Geometry: final body of the model. Coordinates: model frame, mm. Face numbers are marked on the shaded views. A direction names the side the tool comes from. Give positions to 0.01 mm unless a question says otherwise; leave off trailing zeros. Loops run counter-clockwise (first coordinate to the right, second up) from the corner with the lowest first, then second, coordinate; pieces in that order, holes last. Notation, with made-up numbers: (25, 10.5) - (29, 10.5) arc R15 ccw to (29, 27.5) - close; hole circle Ø6 at (-20.5, -34). An arc over 180 degrees is marked (long way). Use one line per item in the form item = value.
```python
from build123d import *

# Parameters (mm, degrees)
F0_R     = 6.985
F1_DEPTH = 12.7


with BuildPart() as f1:
    # F0 (on Top) → F1 (new body)
    with BuildSketch(Plane.XY):
        with BuildLine():
            ThreePointArc((-3.175, 9.651164), (0, 10.16), (3.175, 9.651164))
            Line((3.175, 9.651164), (3.175, 24.243791))
            Line((3.175, 24.243791), (1.5875, 24.243791))
            Line((1.5875, 24.243791), (1.5875, 11.548717))
            Line((1.5875, 11.548717), (-1.5875, 11.548717))
            Line((-1.5875, 11.548717), (-1.5875, 24.243791))
            Line((-1.5875, 24.243791), (-3.175, 24.243791))
            Line((-3.175, 24.243791), (-3.175, 9.651164))
        make_face()
        with BuildLine():
            Line((3.175, 7.733791), (3.175, 9.651164))
            ThreePointArc((3.175, 9.651164), (0, 10.16), (-3.175, 9.651164))
            Line((-3.175, 9.651164), (-3.175, 7.733791))
            Line((-3.175, 7.733791), (3.175, 7.733791))
        make_face()
        with BuildLine():
            Line((7.733791, 3.175), (9.651164, 3.175))
            ThreePointArc((9.651164, 3.175), (7.184205, 7.184205), (3.175, 9.651164))
            Line((3.175, 9.651164), (3.175, 7.733791))
            Line((3.175, 7.733791), (-3.175, 7.733791))
            Line((-3.175, 7.733791), (-3.175, 9.651164))
            ThreePointArc((-3.175, 9.651164), (-7.184205, 7.184205), (-9.651164, 3.175))
            Line((-9.651164, 3.175), (-7.733791, 3.175))
            Line((-7.733791, 3.175), (-7.733791, -3.175))
            Line((-7.733791, -3.175), (-9.651164, -3.175))
            ThreePointArc((-9.651164, -3.175), (-7.184205, -7.184205), (-3.175, -9.651164))
            Line((-3.175, -9.651164), (-3.175, -7.733791))
            Line((-3.175, -7.733791), (3.175, -7.733791))
            Line((3.175, -7.733791), (3.175, -9.651164))
            ThreePointArc((3.175, -9.651164), (7.184205, -7.184205), (9.651164, -3.175))
            Line((9.651164, -3.175), (7.733791, -3.175))
            Line((7.733791, -3.175), (7.733791, 3.175))
        make_face()
        Circle(F0_R, mode=Mode.SUBTRACT)
        with BuildLine():
            ThreePointArc((9.651164, -3.175), (10.031985, -1.607758), (10.16, 0))
            ThreePointArc((10.16, 0), (10.031985, 1.607758), (9.651164, 3.175))
            Line((9.651164, 3.175), (7.733791, 3.175))
            Line((7.733791, 3.175), (7.733791, -3.175))
            Line((7.733791, -3.175), (9.651164, -3.175))
        make_face()
        with BuildLine():
            ThreePointArc((9.651164, 3.175), (10.031985, 1.607758), (10.16, 0))
            ThreePointArc((10.16, 0), (10.031985, -1.607758), (9.651164, -3.175))
            Line((9.651164, -3.175), (24.243791, -3.175))
            Line((24.243791, -3.175), (24.243791, -1.5875))
            Line((24.243791, -1.5875), (11.548717, -1.5875))
            Line((11.548717, -1.5875), (11.548717, 1.5875))
            Line((11.548717, 1.5875), (24.243791, 1.5875))
            Line((24.243791, 1.5875), (24.243791, 3.175))
            Line((24.243791, 3.175), (9.651164, 3.175))
        make_face()
        with BuildLine():
            Line((3.175, -24.243791), (3.175, -9.651164))
            ThreePointArc((3.175, -9.651164), (0, -10.16), (-3.175, -9.651164))
            Line((-3.175, -9.651164), (-3.175, -24.243791))
            Line((-3.175, -24.243791), (-1.5875, -24.243791))
            Line((-1.5875, -24.243791), (-1.5875, -11.548717))
            Line((-1.5875, -11.548717), (1.5875, -11.548717))
            Line((1.5875, -11.548717), (1.5875, -24.243791))
            Line((1.5875, -24.243791), (3.175, -24.243791))
        make_face()
        with BuildLine():
            ThreePointArc((-3.175, -9.651164), (0, -10.16), (3.175, -9.651164))
            Line((3.175, -9.651164), (3.175, -7.733791))
            Line((3.175, -7.733791), (-3.175, -7.733791))
            Line((-3.175, -7.733791), (-3.175, -9.651164))
        make_face()
        with BuildLine():
            Line((-7.733791, 3.175), (-9.651164, 3.175))
            ThreePointArc((-9.651164, 3.175), (-10.16, 0), (-9.651164, -3.175))
            Line((-9.651164, -3.175), (-7.733791, -3.175))
            Line((-7.733791, -3.175), (-7.733791, 3.175))
        make_face()
        with BuildLine():
            ThreePointArc((-9.651164, -3.175), (-10.16, 0), (-9.651164, 3.175))
            Line((-9.651164, 3.175), (-24.243791, 3.175))
            Line((-24.243791, 3.175), (-24.243791, 1.5875))
            Line((-24.243791, 1.5875), (-11.548717, 1.5875))
            Line((-11.548717, 1.5875), (-11.548717, -1.5875))
            Line((-11.548717, -1.5875), (-24.243791, -1.5875))
            Line((-24.243791, -1.5875), (-24.243791, -3.175))
            Line((-24.243791, -3.175), (-9.651164, -3.175))
        make_face()
    extrude(amount=F1_DEPTH)


solid = f1.part
```
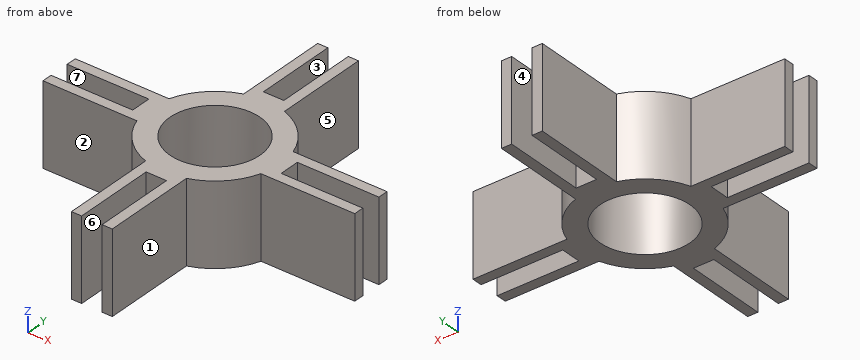
(1) Pin query (flat end, axial travel): P1, Ø6.5, axis at x = 16.5, z = 8, coming from the +Y side (3 decimals); P2, Ø4, axis at y = -10, z = 3.5, coming from the -X side; P3, Ø3, axis at x = 13.5, z = 9, coming from the -Y side (3 decimals). Return the tip coordinate at first contact, or that it passes through.
Solution:
P1 = 3.175
P2 = -6.26
P3 = -3.175
(2) Cut plane A-A (x = -14.5). Return the cut outline in (y, z) (1 decimal).
Solution:
outline = (-3.2, 0) - (-1.6, 0) - (-1.6, 12.7) - (-3.2, 12.7) - close; (1.6, 0) - (3.2, 0) - (3.2, 12.7) - (1.6, 12.7) - close
(3) Pull-direction query (X, two-part tool) for the marked faces 1, 2, 3 and 4; classes: released by +X, released by -X, zero draft, split by the parting line, or undercut.
Solution:
face_1 = released by +X
face_2 = zero draft
face_3 = undercut
face_4 = undercut
(4) Material intervals for L1, parallel to Y at x = 0, z = 8.75 (3 decimals); L2, parallel to Y at x = 14, z = 9.5 (1 decimal), sorted ascending. Write a range as from..to.
Solution:
L1 = -11.549..-6.985, 6.985..11.549
L2 = -3.2..-1.6, 1.6..3.2
(5) Access query for the marked faces 5, 6 and 7. Directions: +Z, -Z, +X, -X, +Y, -Y. A direction counts if a zero-diameter tool reaches every point of the face in a straight line with its end or side. Return the directions, or none.
Solution:
face_5 = +Z, -Z, +X, +Y
face_6 = +Z, -Z, -Y
face_7 = +Z, -Z, -X
(6) Cut plane D-D (y = -10.5). Return the cut outline in (x, z) (3 decimals).
Solution:
outline = (-3.175, 0) - (3.175, 0) - (3.175, 12.7) - (-3.175, 12.7) - close
